from build123d import *

# Parameters (mm, degrees)
F0_R     = 1.5
F0_R_2   = 2.5
F0_W     = 49.869843
F0_H     = 40.004894
F0_W_2   = 30
F0_H_2   = 9
F1_DEPTH = 1.016
F2_DEPTH = 10


with BuildPart() as f1:
    # F0 (on Top) → F1 (new body)
    with BuildSketch(Plane.XY):
        Polygon((0, 53), (0, 0), (14.124727, 0), (14.124727, 9), (44.124727, 9), (44.124727, 0), (129, 0), (129, 53), align=None)
        with Locations((3.492343, 4.177653)):
            Circle(F0_R, mode=Mode.SUBTRACT)
        with Locations((124.5, 7.541248)):
            Circle(F0_R_2, mode=Mode.SUBTRACT)
        with Locations((93.68017, 25.918216)):
            Rectangle(F0_W, F0_H, mode=Mode.SUBTRACT)
        with Locations((124.5, 25.076802)):
            Circle(F0_R_2, mode=Mode.SUBTRACT)
        with Locations((124.5, 43.574877)):
            Circle(F0_R_2, mode=Mode.SUBTRACT)
        with Locations((125.5, 50.5)):
            Circle(F0_R, mode=Mode.SUBTRACT)
        with Locations((93.68017, 25.918216)):
            Rectangle(F0_W, F0_H)
        with Locations((29.124727, 4.5)):
            Rectangle(F0_W_2, F0_H_2)
    extrude(amount=-F1_DEPTH)

    # F0 (on Top) → F2 (join)
    with BuildSketch(Plane.XY):
        with Locations((29.124727, 4.5)):
            Rectangle(F0_W_2, F0_H_2)
        with Locations((93.68017, 25.918216)):
            Rectangle(F0_W, F0_H)
    extrude(amount=F2_DEPTH)


solid = f1.part
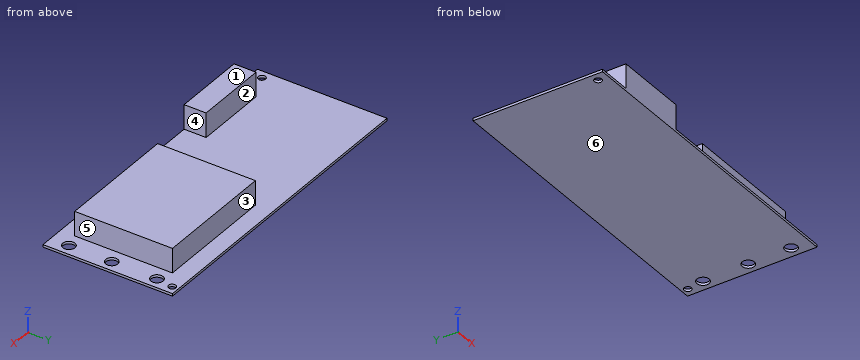
Design review of the part built by this model. Coordinates are the model's own, in mm. Face numbers are marked on the shaded views. A direction names the side the tool comes from. Coordinates: 2 decimals unless noted, no trailing zeros. Loops run counter-clockwise (first coordinate to the right, second up) from the corner with the lowest first, then second, coordinate; pieces in that order, holes last. Notation, with made-up numbers: (26.25, 85.25) -> (81.25, 85.25) arc R34 ccw to (81.25, 117.25) -> close; hole circle Ø1 at (62, 77.5). An arc over 180 degrees is marked (long way). Use a Markdown table: item, result. Add a question column.
Item 1: We need section C-C, the plane y = 50.5. Write out the cut boundary in (x, z), and give its area (3 significant figures).
Item 2: We need section D-D, the plane y = 38.5. Write out the cut boundary in (x, z).
Item 3: The part is to be moulded in two halves that separate along X. For the marked faces 4, 5 and 6, say which applies: +X half, -X half, draft (parallel to the pull), parting line (faces both ways), or undercut.
Item 4: Wall thickness on L1, parallel to Y at x = 124.5, z = -0.55; L2, parallel to Y at x = 125.5, z = -0.45; L3, parallel to X at y = 6, z = 8.5: over which ranges is each line inside the solid? List them lowest first. Write a range as from..to.
Item 5: Clearance check with flat-ended pins moving along their axes: P1, Ø3, axis at x = 96.5, z = 3.5, coming from the +Y side; P2, Ø1, axis at x = 48.5, y = 47.5, coming from the +Z side; P3, Ø2.5, axis at y = 3, z = 4, coming from the +X side; P4, Ø5, axis at x = 125.5, y = 50.5, coming from the -Z side. State where each tip first meets the part, or that it passes through.
Item 6: Machinability: for the marked faces 1, 2 and 3, which of the approach directions +Z, -Z, +X, -X, +Y, -Y give a long, thin tool a straight path to every point of the face, cutting with its end or side? Answer none if there is none.
Item 7: We need section A-A, the plane z = 1.25. Write out the cut boundary in (x, y).
Item 8: We need section B-B, the plane x = 125.5. Write out the cut boundary in (y, z), and give its area (3 significant figures).
Numbers:
| question | item | result |
|---|---|---|
| 1 | outline | (0, -1.02) -> (124, -1.02) -> (124, 0) -> (0, 0) -> close; (127, -1.02) -> (129, -1.02) -> (129, 0) -> (127, 0) -> close |
| 1 | area | 128 mm^2 |
| 2 | outline | (0, -1.02) -> (129, -1.02) -> (129, 0) -> (118.62, 0) -> (118.62, 10) -> (68.75, 10) -> (68.75, 0) -> (0, 0) -> close |
| 3 | face 4 | undercut |
| 3 | face 5 | +X half |
| 3 | face 6 | draft |
| 4 | L1 | y = 0..5.04, 10.04..22.58, 27.58..41.07, 46.07..49.38, 51.62..53 |
| 4 | L2 | y = 0..5.25, 9.83..22.79, 27.37..41.28, 45.87..49, 52..53 |
| 4 | L3 | x = 14.12..44.12, 68.75..118.62 |
| 5 | P1 | stops at y = 45.92 |
| 5 | P2 | stops at z = 0 |
| 5 | P3 | stops at x = 44.12 |
| 5 | P4 | stops at z = -1.02 |
| 6 | face 1 | +Z, +X, -X, +Y, -Y |
| 6 | face 2 | +Z, -X, +Y |
| 6 | face 3 | +Z, +X, -X, +Y |
| 7 | outline | (14.12, 0) -> (44.12, 0) -> (44.12, 9) -> (14.12, 9) -> close; (68.75, 5.92) -> (118.62, 5.92) -> (118.62, 45.92) -> (68.75, 45.92) -> close |
| 8 | outline | (0, -1.02) -> (5.25, -1.02) -> (5.25, 0) -> (0, 0) -> close; (9.83, -1.02) -> (22.79, -1.02) -> (22.79, 0) -> (9.83, 0) -> close; (27.37, -1.02) -> (41.28, -1.02) -> (41.28, 0) -> (27.37, 0) -> close; (45.87, -1.02) -> (49, -1.02) -> (49, 0) -> (45.87, 0) -> close; (52, -1.02) -> (53, -1.02) -> (53, 0) -> (52, 0) -> close |
| 8 | area | 36.8 mm^2 |
